Here's how the part is built. I have some questions about the finished solid (model axes, mm). Coordinates: 2 decimals unless noted, no trailing zeros. Write each loop counter-clockwise with the first axis right and the second up, starting at its lowest first coordinate (ties: lowest second). Pieces come first, ordered by that corner, then holes.
Item 1: If I drill on line 1 (Y direction, x = 5.5, z = 134.5); line 2 (X direction, y = -7.5, z = 147), over which ranges is the centre line in solid material (lowest first)?
Item 2: If we section it at B-B (x = -2.5): Please give me the cut outline in (y, z).
Item 3: If we section it at A-A (y = 2.5): Please give me the cut outline in (x, z).
Item 4: If we section it at C-C (z = 101): Please give me the cut outline in (x, y), then the cut area to 3 significant figures.
Autodesk Inventor part; units mm, degrees
ref_plane "Start Plane" through (0, 0, 4.614) normal (0, 0, 1) x (1, 0, 0)
ref_plane "End Plane" through (0, 0, 255.3168) normal (0, 0, 1) x (1, 0, 0)
ref_plane "Work Plane4" through (10.1657, 0, 255.4635) normal (-0.6628, 0, 0.7488) x (0.7488, 0, 0.6628)
ref_plane "Start Plane" through (0, 0, 4.614) normal (0, 0, 1) x (1, 0, 0)
ref_plane "End Plane" through (0, 0, 255.3168) normal (0, 0, 1) x (1, 0, 0)
sketch "Sketch" plane through (0, 0, 0) normal (0, 0, 1) x (1, 0, 0)
  line L0 (-10, -7) -> (-10, 7)
  line L1 (-7, 10) -> (7, 10)
  line L2 (10, 7) -> (10, -7)
  line L3 (7, -10) -> (-7, -10)
  arc A0 (-10, -7) -> (-7, -10) centre (-7, -7) ccw
  arc A1 (-7, 10) -> (-10, 7) centre (-7, 7) ccw
  arc A2 (10, 7) -> (7, 10) centre (7, 7) ccw
  arc A3 (7, -10) -> (10, -7) centre (7, -7) ccw
  arc A4 (-7, 8) -> (-8, 7) centre (-7, 7) ccw
  line L4 (-7, 8) -> (7, 8)
  arc A5 (8, 7) -> (7, 8) centre (7, 7) ccw
  line L5 (8, 7) -> (8, -7)
  arc A6 (7, -8) -> (8, -7) centre (7, -7) ccw
  line L6 (7, -8) -> (-7, -8)
  arc A7 (-8, -7) -> (-7, -8) centre (-7, -7) ccw
  line L7 (-8, -7) -> (-8, 7)
  line L8 (0, 14.8698) -> (0, -14.8698) construction
  line L9 (-14.8698, 0) -> (14.8698, 0) construction
  dimension "d7" = 3
  dimension "d10" = 20
  dimension "d11" = 20
  dimension "d12" = 2
  dimension "d15" = 10
  dimension "d16" = 10
extrude "Body" add sketch "Sketch" along normal up to surface (250.7028 mm away) from surface at 4.614
sketch "Sketch3" plane through (0, 0, 0) normal (0, 0, 1) x (1, 0, 0)
  line L0 (0, 0) -> (10, 0)
ref_plane "Work Plane3" through (0, 0, 0) normal (0, -1, 0) x (1, 0, 0)
sketch "Sketch4" plane through (0, 0, 0) normal (0, -1, 0) x (1, 0, 0)
  line L0 (-2, 4.614) -> (12, 4.614)
  line L1 (-2, 255.3168) -> (12, 255.3168)
  dimension "d18" = 250.7028
ref_plane "Work Plane4" through (10.1657, 0, 255.4635) normal (-0.6628, 0, 0.7488) x (0.7488, 0, 0.6628)
split "Split1" plane through (10.1657, 0, 255.4635) removes the side toward (-0.6628, 0, 0.7488)
ref_plane "Work Plane8" through (-138.1713, -4.0763, 306.3066) normal (0.3124, 0.267, 0.9117) x (0.949, -0.0436, -0.3124)
split "Split2" plane through (-138.1713, -4.0763, 306.3066) removes the side toward (0.3124, 0.267, 0.9117)
ref_plane "Work Plane9" through (-4.1619, 10.0613, 9.4487) normal (-0.3124, -0.267, -0.9117) x (-0.1048, -0.9442, 0.3124)
split "Split3" plane through (-4.1619, 10.0613, 9.4487) removes the side toward (-0.3124, -0.267, -0.9117)
equation "\"d7\" = G_IR"
equation "\"d10\" = G_H"
equation "\"d11\" = G_W"
equation "\"d12\" = G_T"
equation "\"d15\" = 0.5 * d10"
equation "\"d16\" = 0.5 * d11"
equation "\"d3\" = G_L"
equation "\"G_W\" = 20"
equation "\"G_H\" = 20"
equation "\"G_T\" = 2"
equation "\"G_IR\" = 3"
equation "\"G_L\" = 250.12582"
equation "\"G_OFFSET_START\" = -4.61403"
equation "\"G_OFFSET_END\" = 8.51725"
equation "\"d13\" = -G_OFFSET_START"
equation "\"d14\" = G_OFFSET_END + B_L"
equation "\"B_L\" = 246.79957"
properties part number "ISO 12633-2 - 20x20x2 - 250,13" material "Steel, Mild"
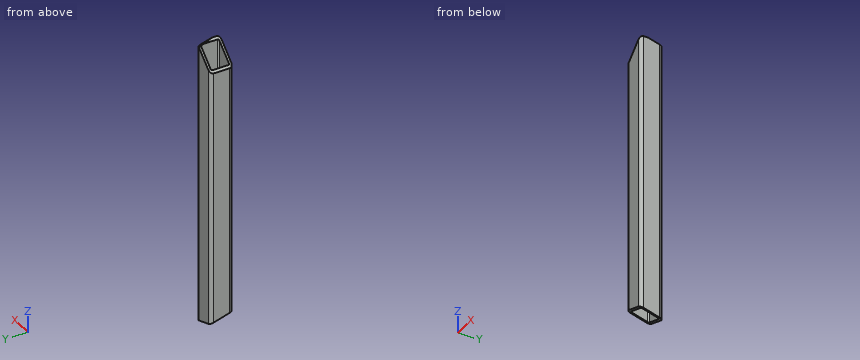
Answer list:
1. line 1: y = -10 to -8, 8 to 10
1. line 2: x = -9.96 to -7.87, 7.87 to 9.96
2. outline: (-10, 14.75) - (-8, 14.17) - (-8, 244.25) - (-10, 244.25) - close; (8, 9.48) - (10, 8.9) - (10, 244.25) - (8, 244.25) - close
3. outline: (-10, 13.66) - (-8, 12.98) - (-8, 239.38) - (-10, 237.61) - close; (8, 7.5) - (10, 6.81) - (10, 253.61) - (8.61, 254.09) - (8, 253.55) - close
4. outline: (-10, -7) arc R3 ccw to (-7, -10) - (7, -10) arc R3 ccw to (10, -7) - (10, 7) arc R3 ccw to (7, 10) - (-7, 10) arc R3 ccw to (-10, 7) - close; hole (-8, -7) arc R1 ccw to (-7, -8) - (7, -8) arc R1 ccw to (8, -7) - (8, 7) arc R1 ccw to (7, 8) - (-7, 8) arc R1 ccw to (-8, 7) - close
4. area: 137 mm2
